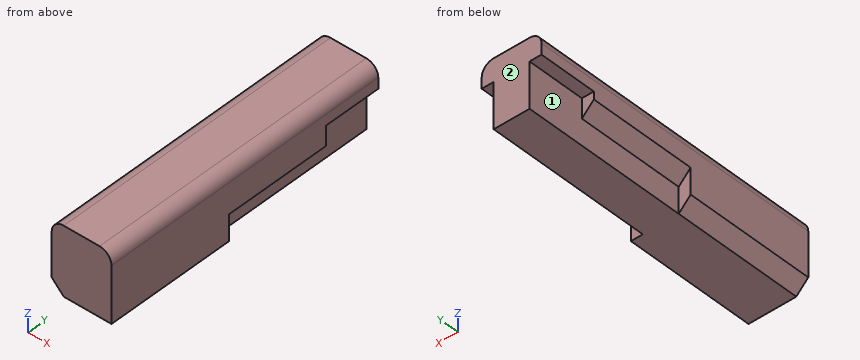
```python
from build123d import *

# Parameters (mm, degrees)
F1_DEPTH  = 25.4
F2_R      = 5.08
F3_R      = 5.08
F4_SIZE   = 5.08
F5_R      = 6.332586
F1_FACE_W = 15.24
F1_FACE_H = 125.814986
F6_DEPTH  = 28.999906


with BuildPart() as f1:
    # F0 (on Right) → F1 (new body)
    with BuildSketch(Plane.YZ):
        Polygon((70.343368, 0), (-55.471618, 0), (-55.471618, -28.999906), (0, -28.999906), (0, -17.994815), (45.656264, -17.994815), (45.656264, -9.666636), (70.343368, -9.666636), align=None)
    extrude(amount=F1_DEPTH)

    # F2
    f2_edges = [f1.edges().sort_by_distance(p)[0] for p in [
        (25.4, 7.435875, 0),
    ]]
    fillet(f2_edges, radius=F2_R)

    # F3
    f3_edges = [f1.edges().sort_by_distance(p)[0] for p in [
        (0, 7.435875, 0),
    ]]
    fillet(f3_edges, radius=F3_R)

    # F4
    f4_edges = [f1.edges().sort_by_distance(p)[0] for p in [
        (0, -27.735809, -28.999906),
        (0, 22.828132, -17.994815),
    ]]
    chamfer(f4_edges, length=F4_SIZE)

    # F5 (on Top) + F1_face (on face) → F6 (join, through all)
    with BuildSketch(Plane.XY):
        with Locations((12.965518, 0)):
            Circle(F5_R)
    with BuildSketch(Plane(origin=(12.7, 7.435875, 0), x_dir=(1, 0, 0), z_dir=(0, 0, 1))):
        Rectangle(F1_FACE_W, F1_FACE_H)
    extrude(amount=-F6_DEPTH)


solid = f1.part
```
The listing builds one solid part. Answer for the finished solid, in the listing's coordinates (mm). Face numbers are marked on the shaded views. A direction names the side the tool comes from. Round coordinates to 2 decimals unless told otherwise and drop trailing zeros. Loops run counter-clockwise (first coordinate to the right, second up) from the corner with the lowest first, then second, coordinate; pieces in that order, holes last. Notation, with made-up numbers: (46.5, 53.5) - (104.5, 53.5) arc R18 ccw to (104.5, 79.5) - close; hole circle Ø5 at (-18.5, 29). An arc over 180 degrees is marked (long way). Use one line per item in the form item = value. Start each with the question number.
1. The part is cut by section D-D on y = -33. Determine the outline of the cut face in (x, z).
2. A tool of negligible diameter and unlimited length cuts with its end or side. For the marked faces 1 and 2, from which of +Z, -Z, +X, -X, +Y, -Y can it reach the whole face along a straight path? Write none if from no direction.
3. Given pin 1 Ø1 at (y, z) = (-34.5, -4) entering from -X; pin 2 Ø5.5 at (x, z) = (3, -13) entering from +Y; pin 3 Ø1.5 at (y, z) = (38.5, -26) entering from -X; pin 4 Ø3 at (y, z) = (-23, -26) entering from -X, each flat-ended and moving along its own axis, determine where each tip first touches the part or whether it passes through.
4. The part is cut by section A-A on y = 55. Determine the outline of the cut face in (x, z), then the cut area to 3 significant figures.
5. The part is cut by section C-C on x = 22.75. Determine the outline of the cut face in (y, z), then the cut area to 3 significant figures.
6. Consider line 1 (X direction, y = 50.5, z = -16.75); line 2 (Y direction, x = 2.5, z = -16.25); line 3 (Y direction, x = 3.5, z = -10). Determine where each line is inside the solid, lowest interval first. Write a range as [from, to].
7. The part is cut by section B-B on z = -10.75. Determine the outline of the cut face in (x, y), then the cut area to 3 significant figures.
Geometry check:
q1.outline = (0, -23.92) - (5.08, -29) - (25.4, -29) - (25.4, -5.08) arc R5.08 ccw to (20.32, 0) - (5.08, 0) arc R5.08 ccw to (0, -5.08) - close
q2.face_1 = -Z, -X, +Y
q2.face_2 = +Z, -Z, +X, -X, +Y
q3.pin_1 = 0.03
q3.pin_2 = 70.34
q3.pin_3 = 5.08
q3.pin_4 = 0.58
q4.outline = (0, -9.67) - (5.08, -9.67) - (5.08, -29) - (20.32, -29) - (20.32, -9.67) - (25.4, -9.67) - (25.4, -5.08) arc R5.08 ccw to (20.32, 0) - (5.08, 0) arc R5.08 ccw to (0, -5.08) - close
q4.area = 529 mm^2
q5.outline = (-55.47, -29) - (0, -29) - (0, -17.99) - (45.66, -17.99) - (45.66, -9.67) - (70.34, -9.67) - (70.34, -0.62) - (-55.47, -0.62) - close
q5.area = 2,590 mm^2
q6.line_1 = [5.08, 20.32]
q6.line_2 = [-55.47, 0]
q6.line_3 = [-55.47, 45.66]
q7.outline = (0, -55.47) - (25.4, -55.47) - (25.4, 45.66) - (20.32, 45.66) - (20.32, 70.34) - (5.08, 70.34) - (5.08, 45.66) - (0, 45.66) - close
q7.area = 2,940 mm^2
